Geometry: final body of the model. Coordinates: model frame, mm. A direction names the side the tool comes from. Round coordinates to 2 decimals unless told otherwise and drop trailing zeros. Order: outer loops, then holes, each group sorted by start corner. A loop starts at its lowest first (then second) coordinate and runs counter-clockwise, first axis right, second up. Notation, with made-up numbers: (-8.5, -11) - (26.5, -11) arc R20 cw to (26.5, 24) - close; hole circle Ø3 at (-12.5, -9). An arc over 180 degrees is marked (long way). Put each result on its own line as item: value. Start each with the question number.
(1) Access query for faces 1 (the face through (-1, -60, 14)), 2 (the face through (-1, 1, 7)). Directions: +Z, -Z, +X, -X, +Y, -Y. A direction counts if a zero-diameter tool reaches every point of the face in a straight line with its end or side. Return the directions, or none.
(2) Section C-C (y = 9.5). Output: boundary loops of the cut face in (x, z).
(3) Pull-direction query (X, two-part tool) for faces 3 (the face through (-1, 60, 14)), 4 (the face through (-0.65, 34.71, 3.55)), 5 (the face through (60, -1, 14)); classes: released by +X, released by -X, zero draft, split by the parting line, or undercut.
(4) Section A-A (x = 0). Output: boundary loops of the cut face in (y, z), and give its area (3 significant figures).
(5) Material intervals for L1, parallel to X at y = 20.5, z = 27.5; L2, parallel to Y at x = 0, z = 4.5, sorted ascending. Write a range as [from, to].
(6) Pin query (flat end, axial travel): P1, Ø8, axis at x = 0, y = 37.64, coming from the -Z side; P2, Ø5, axis at x = 31, y = -22.5, coming from the +Z side. Return the tip coordinate at first contact, or that it passes through.
(7) Section B-B (z = 26.5). Output: boundary loops of the cut face in (x, y).
from build123d import *

# Parameters (mm, degrees)
F0_W     = 120
F0_H     = 120
F1_DEPTH = 29
F2_T     = -7
F3_R     = 1.25
F4_DEPTH = 4
F5_R     = 3
F6_DEPTH = 7


with BuildPart() as f1:
    # F0 (on Top) → F1 (new body)
    with BuildSketch(Plane.XY):
        Rectangle(F0_W, F0_H)
    extrude(amount=F1_DEPTH)

    # F2
    f2_openings = [f1.faces().sort_by_distance(p)[0] for p in [
        (0, 0, 29),
    ]]
    offset(amount=F2_T, openings=f2_openings)

    # F3 (on face) → F4 (join)
    with BuildSketch(Plane.XY.offset(29)):
        with BuildLine():
            ThreePointArc((-55, 56.25), (-55.883883, 54.116117), (-53.75, 55))
            ThreePointArc((-53.75, 55), (-54.116117, 55.883883), (-55, 56.25))
        make_face()
        with Locations((55, 55)):
            Circle(F3_R)
        with Locations((55, -55)):
            Circle(F3_R)
        with Locations((-55, -55)):
            Circle(F3_R)
    extrude(amount=F4_DEPTH)

    # F5 (on face) → F6 (cut)
    with BuildSketch(Plane.XY.offset(7)):
        with Locations((0, 37.63944)):
            Circle(F5_R)
    extrude(amount=-F6_DEPTH, mode=Mode.SUBTRACT)


solid = f1.part
Checks:
1. face 1: +Z, -Z, +X, -X, -Y
1. face 2: +Z
2. outline: (-60, 0) - (60, 0) - (60, 29) - (53, 29) - (53, 7) - (-53, 7) - (-53, 29) - (-60, 29) - close
3. face 3: zero draft
3. face 4: undercut
3. face 5: released by +X
4. outline: (-60, 0) - (34.64, 0) - (34.64, 7) - (-53, 7) - (-53, 29) - (-60, 29) - close; (40.64, 0) - (60, 0) - (60, 29) - (53, 29) - (53, 7) - (40.64, 7) - close
4. area: 1,110 mm²
5. L1: x = [-60, -53], [53, 60]
5. L2: y = [-60, 34.64], [40.64, 60]
6. P1: stops at z = 0
6. P2: stops at z = 7
7. outline: (-60, -60) - (60, -60) - (60, 60) - (-60, 60) - close; hole (-53, -53) - (53, -53) - (53, 53) - (-53, 53) - close
